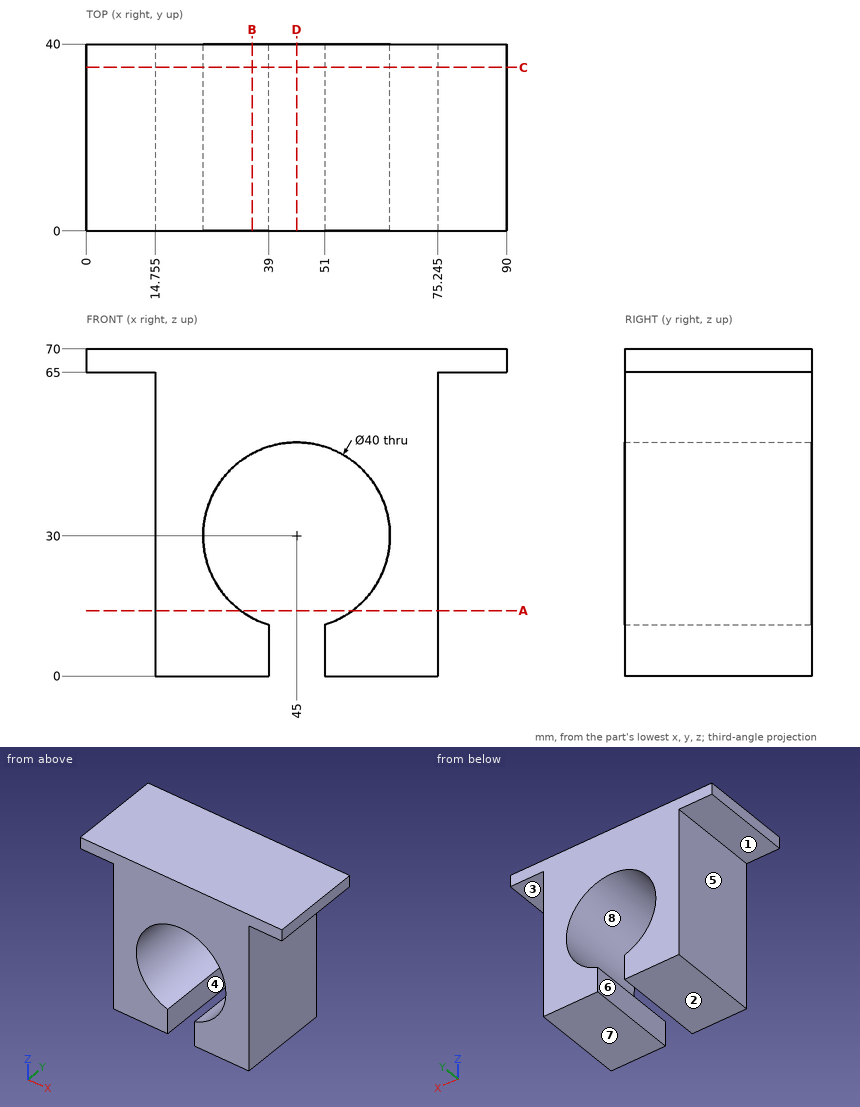
Can you work these out from the drawing? Everything is in mm from the part's minimum corner. A direction names the side the tool comes from. Give positions to 0.01 mm unless a question says otherwise; leave off trailing zeros. Loops run counter-clockwise (first coordinate to the right, second up) from the corner with the lowest first, then second, coordinate; pieces in that order, holes last. Notation, with made-up numbers: (7, 20.5) - (42, 20.5) arc R10 ccw to (42, 34.5) - close; hole circle Ø4 at (-2, 38). An arc over 180 degrees is marked (long way). Answer as a JSON object with one key per item and string values.
Q1. Will these pins go through, and if not, where does the flat tip stop? P1, Ø7.5, axis at x = 82, y = 25, coming from the -Z side; P2, Ø6, axis at x = 79.5, z = 22.5, coming from the -Y side; P3, Ø1.5, axis at x = 41.5, y = 14, coming from the -Z side; P4, Ø12, axis at y = 18.5, z = 17, coming from the +X side (1 decimal).
Geometry says:
{"P1": "z = 65", "P2": "through", "P3": "z = 49.54", "P4": "x = 75.2"}
Q2. Imagine slicing it at A-A on z = 14. Write out the boundary of the cut face in (x, y) (1 decimal), plus the area to 3 significant figures.
Geometry says:
{"outline": "(14.8, 0) - (33, 0) - (33, 40) - (14.8, 40) - close; (57, 0) - (75.2, 0) - (75.2, 40) - (57, 40) - close", "area": "1,460 mm²"}
Q3. Imagine slicing it at C-C on y = 35. Write out the boundary of the cut face in (x, z) (1 decimal).
Geometry says:
{"outline": "(0, 65) - (14.8, 65) - (14.8, 0) - (39, 0) - (39, 10.9) arc R20 cw (long way) to (51, 10.9) - (51, 0) - (75.2, 0) - (75.2, 65) - (90, 65) - (90, 70) - (0, 70) - close"}
Q4. If I drill on L1, parallel to X at y = 14, z = 30 (1 decimal); L2, parallel to Z at x = 14, y = 27; L3, parallel to Z at x = 52, y = 6 (1 decimal), over which ranges is the centre line in solid material (lowest first)?
Geometry says:
{"L1": "14.8 to 25, 65 to 75.2", "L2": "65 to 70", "L3": "0 to 11.3, 48.7 to 70"}
Q5. Imagine slicing it at B-B on x = 35.5. Write out the boundary of the cut face in (y, z), plus the area to 3 significant figures.
Geometry says:
{"outline": "(0, 0) - (40, 0) - (40, 12.4) - (0, 12.4) - close; (0, 47.6) - (40, 47.6) - (40, 70) - (0, 70) - close", "area": "1,390 mm²"}
Q6. Which directions (+Z, -Z, +X, -X, +Y, -Y) give clear straight access to the entire face, cutting with the end or side of a thin tool? Please do the marked faces 1, 2, 3 and 4.
Geometry says:
{"face 1": "-Z, -X, +Y, -Y", "face 2": "-Z, +X, -X, +Y, -Y", "face 3": "-Z, +X, +Y, -Y", "face 4": "-Z, +Y, -Y"}
Q7. If we mould it in two halves opening along X, with no side actions, what happens to the marked faces 5, 6, 7 and 8? For each: pulls with the +X half, pulls with the -X half, needs draft (parallel to the pull), parting line crosses it, or undercut.
Geometry says:
{"face 5": "pulls with the -X half", "face 6": "undercut", "face 7": "needs draft", "face 8": "undercut"}
Q8. Imagine slicing it at D-D on x = 45. Write out the boundary of the cut face in (y, z).
Geometry says:
{"outline": "(0, 50) - (40, 50) - (40, 70) - (0, 70) - close"}
